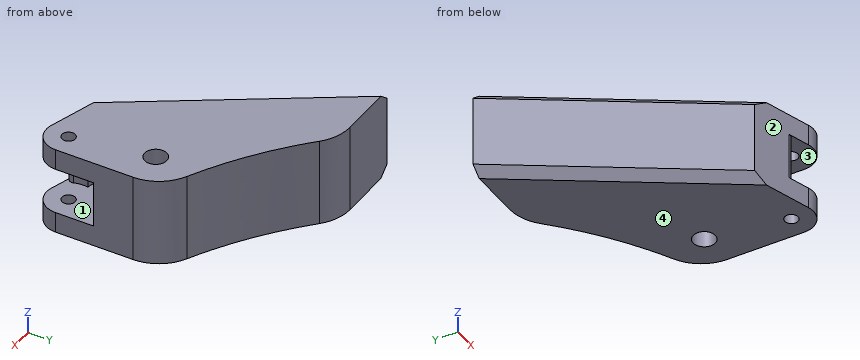
```python
from build123d import *

# Parameters (mm, degrees)
EXTRUDE_1_DEPTH       = 20
FILLET_1_R            = 5
SKETCH_2_R            = 1.5000000000000024
CUT_EXTRUDE_1_DEPTH   = 24
CUT_EXTRUDE_START     = -5
SKETCH_3_R            = 7.5
CUT_EXTRUDE_2_DEPTH   = 10
CHAMFER_1_SIZE        = 2
FILLET_4_R            = 5
SKETCH_5_R            = 2.5000000000000018
CUT_EXTRUDE_3_DEPTH   = 25
EXTRUDE_START         = -11.5
SKETCH_6_R            = 2.5000000000000004
SKETCH_6_R_2          = 1.7499999999999998
EXTRUDE_2_DEPTH       = 3
CUT_EXTRUDE_4_DEPTH   = 34
FILLET_5_R            = 10
FILLET_6_R            = 10
CHAMFER_START         = 15.398006277
CHAMFER_2_OUTLINE_W   = 6.958890637
CHAMFER_2_OUTLINE_H   = 10.000000000000002
CHAMFER_2_DEPTH       = 3.601993723
CHAMFER_START_2       = 14
CHAMFER_2_2_OUTLINE_W = 6.958890637
CHAMFER_2_2_OUTLINE_H = 10.000000000000002
CHAMFER_2_2_DEPTH     = 1.398006277
SKETCH_9_R            = 10.000000000005517
CUT_EXTRUDE_5_DEPTH   = 10
EXTRUDE_4_DEPTH       = 10
FILLET_7_R            = 1
FILLET_8_R            = 10
CUT_EXTRUDE_START_2   = -0.25
CUT_EXTRUDE_6_DEPTH   = 0.25
CUT_EXTRUDE_7_DEPTH   = 0.25


with BuildPart() as part:
    # 草图1 → 凸台-拉伸1 (new body)
    with BuildSketch(Plane.XY):
        Polygon((0, 0), (-26.811555509164208, 22.497566339028918), (-49.8115555091642, 22.49756633902892), (-20.084941781424334, -23.776923785463527), (-0.08494178142433392, -29.999879747988462), align=None)
    extrude(amount=EXTRUDE_1_DEPTH)

    # 圆角1
    fillet_1_edges = [part.edges().sort_by_distance(p)[0] for p in [
        (-0.08494178142433392, -29.999879747988462, 10),
    ]]
    fillet(fillet_1_edges, radius=FILLET_1_R)

    # 草图2 → 切除-拉伸1 (cut)
    with BuildSketch(Plane.XY.offset(20)):
        with Locations((-5.0657473249540095, -23.213671166892293)):
            Circle(SKETCH_2_R)
    extrude(amount=-CUT_EXTRUDE_1_DEPTH, mode=Mode.SUBTRACT)

    # 草图3 → 切除-拉伸2 (cut)
    with BuildSketch(Plane.XY.offset(20).offset(CUT_EXTRUDE_START)):
        with Locations((-5.0657473249540095, -23.213671166892293)):
            Circle(SKETCH_3_R)
    extrude(amount=-CUT_EXTRUDE_2_DEPTH, mode=Mode.SUBTRACT)

    # 倒角1
    chamfer_1_edges = [part.edges().sort_by_distance(p)[0] for p in [
        (-34.94824864529427, -0.6396787232173011, 20),
        (-34.94824864529427, -0.6396787232173011, 0),
    ]]
    chamfer(chamfer_1_edges, length=CHAMFER_1_SIZE)

    # 圆角4
    fillet_4_edges = [part.edges().sort_by_distance(p)[0] for p in [
        (0, 0, 10),
    ]]
    fillet(fillet_4_edges, radius=FILLET_4_R)

    # 草图5 → 切除-拉伸3 (cut)
    with BuildSketch(Plane.XY.offset(20)):
        with Locations((-8.014794077059545, -5.213671166892294)):
            Circle(SKETCH_5_R)
    extrude(amount=-CUT_EXTRUDE_3_DEPTH, mode=Mode.SUBTRACT)

    # 草图6 → 凸台-拉伸2 (add)
    with BuildSketch(Plane(origin=(0, 0, 0), x_dir=(-1, 0, 0), z_dir=(0, 0, -1)).offset(EXTRUDE_START)):
        with Locations(Location((8.014794077059545, -5.213671166892294, 0), (0, 0, 180))):
            Circle(SKETCH_6_R)
        with Locations((8.014794077059545, -5.213671166892294)):
            Circle(SKETCH_6_R_2, mode=Mode.SUBTRACT)
    extrude(amount=EXTRUDE_2_DEPTH)

    # 草图7 → 切除-拉伸4 (cut)
    with BuildSketch(Plane.XY.offset(20)):
        with BuildLine():
            Line((-31.431124160284014, 22.497566339028918), (-26.811555509164208, 22.497566339028918))
            Line((-26.811555509164208, 22.497566339028918), (-1.7926678262045348, 1.5042269117916054))
            add(Edge.make_bspline(
                [(-1.7926678262045348, 1.5042269117916054), (-18.67112927693908, 9.044601568140122), (-31.431124160284014, 22.497566339028918)],
                knots=[0, 0, 0, 1, 1, 1], degree=2))
        make_face()
    extrude(amount=-CUT_EXTRUDE_4_DEPTH, mode=Mode.SUBTRACT)

    # 圆角5
    fillet_5_edges = [part.edges().sort_by_distance(p)[0] for p in [
        (-1.792667826204533, 1.504226911791605, 10),
    ]]
    fillet(fillet_5_edges, radius=FILLET_5_R)

    # 圆角6
    # the kernel refuses this fillet: 10 mm, written as the material it takes off along each edge
    with BuildSketch(Plane(origin=(-11.888995884089002, -26.327074304981263, 5), x_dir=(-0.9548468391902787, 0.29709849156186213, 0), z_dir=(0, 0, 1))) as fillet_6_piece_1:
        with BuildLine():
            CenterArc((11.180339887498954, -9.999999999999998), FILLET_6_R, 90.00000000000001, 73.39845040097977)
            ThreePointArc((1.597191412499857, -7.142857142857143), (1.7290806033645267, -3.3633658232300525), (0, 0))
            Line((0, 0), (11.180339887498953, -2e-17))
        make_face()
    extrude(amount=10, mode=Mode.SUBTRACT)

    # 倒角2: read off the stored shape, not the designer's step
    # 倒角2 outline → 倒角2 (cut)
    with BuildSketch(Plane(origin=(0, 0, 0), x_dir=(0.9972181140668777, 0.0745388018209292, 0), z_dir=(0.07453880182092919, -0.9972181140668778, 0)).offset(CHAMFER_START)):
        with Locations((-4.674246913499999, 10)):
            Rectangle(CHAMFER_2_OUTLINE_W, CHAMFER_2_OUTLINE_H)
    extrude(amount=CHAMFER_2_DEPTH, mode=Mode.SUBTRACT)

    # Chamfer 2 2 outline → Chamfer 2 2 (add)
    with BuildSketch(Plane(origin=(0, 0, 0), x_dir=(0.9972181140668777, 0.0745388018209292, 0), z_dir=(0.07453880182092919, -0.9972181140668778, 0)).offset(CHAMFER_START_2)):
        with Locations((-4.674246913499999, 10)):
            Rectangle(CHAMFER_2_2_OUTLINE_W, CHAMFER_2_2_OUTLINE_H)
    extrude(amount=CHAMFER_2_2_DEPTH)

    # 草图9 → 切除-拉伸5 (cut)
    with BuildSketch(Plane.XY.offset(4.999999999999999)):
        with Locations((-5.065747324960373, -23.21367116689012)):
            Circle(SKETCH_9_R)
    extrude(amount=CUT_EXTRUDE_5_DEPTH, mode=Mode.SUBTRACT)

    # 草图10 → 凸台-拉伸4 (add)
    with BuildSketch(Plane.XY.offset(4.999999999999999)):
        with BuildLine():
            Line((-20.306861182467813, -23.431468792638793), (-20.084941781424334, -23.776923785463527))
            Line((-20.084941781424334, -23.776923785463527), (-8.739068741608744, -27.30716719962209))
            ThreePointArc((-8.739068741608744, -27.30716719962209), (-10.29932188852527, -24.904735118255193), (-10.439836916118015, -22.04355960545204))
            Line((-10.439836916118015, -22.04355960545204), (-14.836819308888755, -21.086195600637897))
            ThreePointArc((-14.836819308888755, -21.086195600637897), (-14.95313679387356, -21.717165406749196), (-15.028752577744056, -22.354295618532444))
            ThreePointArc((-15.028752577744056, -22.354295618532444), (-17.59390852193624, -23.254981419998394), (-20.306861182467813, -23.431468792638793))
        make_face()
    extrude(amount=EXTRUDE_4_DEPTH)

    # 圆角7
    fillet_7_edges = [part.edges().sort_by_distance(p)[0] for p in [
        (-8.739068741608744, -27.30716719962209, 10),
    ]]
    fillet(fillet_7_edges, radius=FILLET_7_R)

    # 圆角8
    fillet_8_edges = [part.edges().sort_by_distance(p)[0] for p in [
        (-31.431124160284014, 22.497566339028918, 10),
    ]]
    fillet(fillet_8_edges, radius=FILLET_8_R)

    # 草图11 → 切除-拉伸6 (cut)
    with BuildSketch(Plane(origin=(0, 0, 15), x_dir=(-1, 0, 0), z_dir=(0, 0, -1)).offset(CUT_EXTRUDE_START_2)):
        with BuildLine():
            Line((6.551239782763319, -27.987905362843687), (11.44337405787706, -26.4657285550041))
            ThreePointArc((11.44337405787706, -26.4657285550041), (10.418424754087408, -26.19661722979815), (10.210809683029842, -25.157464708287105))
            ThreePointArc((10.210809683029842, -25.157464708287105), (10.550931066650136, -23.617105572837715), (10.439836916118015, -22.04355960545204))
            Line((10.439836916118015, -22.04355960545204), (14.836819308888755, -21.086195600637897))
            ThreePointArc((14.836819308888755, -21.086195600637897), (9.097555674937517, -14.06246788922412), (0.04124678677052372, -14.567608806379399))
            Line((0.04124678677052372, -14.567608806379399), (0.06576736695593181, -23.227828130463013))
            ThreePointArc((0.06576736695593181, -23.227828130463013), (2.1072866759334765, -27.24449125568279), (6.551239782763319, -27.987905362843687))
        make_face()
    extrude(amount=CUT_EXTRUDE_6_DEPTH, mode=Mode.SUBTRACT)

    # 草图12 → 切除-拉伸7 (cut)
    with BuildSketch(Plane.XY.offset(4.999999999999999)):
        with BuildLine():
            Line((-14.836819308888755, -21.086195600637897), (-10.439836916118015, -22.04355960545204))
            ThreePointArc((-10.439836916118015, -22.04355960545204), (-10.550931066650133, -23.617105572837712), (-10.21080968302984, -25.157464708287105))
            ThreePointArc((-10.21080968302984, -25.157464708287105), (-10.418424754087408, -26.19661722979815), (-11.44337405787706, -26.465728555004105))
            Line((-11.44337405787706, -26.465728555004105), (-6.551239782763319, -27.987905362843687))
            ThreePointArc((-6.551239782763319, -27.987905362843687), (-2.107286675933478, -27.24449125568279), (-0.06576736695593308, -23.227828130463013))
            Line((-0.06576736695593308, -23.227828130463013), (-0.04124678677052488, -14.567608806379397))
            ThreePointArc((-0.04124678677052488, -14.567608806379397), (-9.097555674937517, -14.062467889224122), (-14.836819308888755, -21.086195600637897))
        make_face()
    extrude(amount=-CUT_EXTRUDE_7_DEPTH, mode=Mode.SUBTRACT)


solid = part.part
```
CAD build for the part. Positions are in the model's coordinates, mm. Face numbers are marked on the shaded views. Coordinates: 2 decimals unless noted, no trailing zeros. Order: outer loops, then holes, each group sorted by start corner. A loop starts at its lowest first (then second) coordinate and runs counter-clockwise, first axis right, second up. Notation, with made-up numbers: (-12, 4.25) - (38, 4.25) arc R28 ccw to (38, 29.25) - close; hole circle Ø7 at (-37.75, 54.25). An arc over 180 degrees is marked (long way). Answer in a Markdown table with one row per item.
1. Slice it at C-C, the plane y = -12. List the corners of the cut face in (x, z), then the cut area to 3 significant figures.
Answer:
| item | result |
|---|---|
| outline | (-27.65, 2) - (-25.27, 0) - (-0.03, 0) - (-0.03, 20) - (-25.27, 20) - (-27.65, 18) - close |
| area | 548 mm² |
2. Flat gauge pins, fed straight in: P1, Ø3, axis at x = -33.5, z = 11, coming from the +Y side; P2, Ø1.5, axis at x = -19.5, z = 15.5, coming from the -Y side; P3, Ø10, axis at y = -20, z = 3, coming from the +X side. Where does each tip first touch, or does it go through?
Answer:
| item | result |
|---|---|
| P1 | y = 22.48 |
| P2 | y = -24.19 |
| P3 | x = -0.04 |
3. Slice it at A-A, the plane x = -40. List the corners of the cut face in (y, z).
Answer:
| item | result |
|---|---|
| outline | (7.22, 2) - (10.92, 0) - (22.5, 0) - (22.5, 20) - (10.92, 20) - (7.22, 18) - close |
4. Pull direction Z, two halves, no side cores. Call the marked faces 1, 2, 3 and 4: +Z half, -Z half, draft (parallel to the pull), parting line (faces both ways), or undercut.
Answer:
| item | result |
|---|---|
| face 1 | undercut |
| face 2 | draft |
| face 3 | undercut |
| face 4 | -Z half |
5. Drill centre lines: L1, parallel to X at y = -6, z = 16; L2, parallel to X at y = -14, z = 5.75; L3, parallel to Y at x = -29, z = 8.75. Where is each one in solid material? Low to high. Write a range as from..to.
Answer:
| item | result |
|---|---|
| L1 | -31.5..-10.39, -5.64..-0.02 |
| L2 | -26.37..-8.95, -1.18..-0.04 |
| L3 | -9.9..20.01 |
6. Slice it at B-B, the plane z = 16. Give the number of separate pieces and of enclosed holes in the cut face, then the cut area to 3 significant figures.
Answer:
| item | result |
|---|---|
| separate pieces | 1 |
| enclosed holes | 2 |
| area | 1,240 mm² |
